from build123d import *

# Parameters (mm, degrees)
BOSS_EXTRUDE1_DEPTH                               = 20
CSK_FOR_3_FLAT_HEAD_MACHINE_SCREW_100_D           = 2.794
CSK_FOR_3_FLAT_HEAD_MACHINE_SCREW_100_DEPTH       = 20
CSK_FOR_3_FLAT_HEAD_MACHINE_SCREW_100_CSINK_D     = 5.0546
CSK_FOR_3_FLAT_HEAD_MACHINE_SCREW_100_CSINK_ANGLE = 100


with BuildPart() as part:
    # Sketch2 → Boss-Extrude1 (new body)
    with BuildSketch(Plane.XY):
        Polygon((-118.58, 345.487717935), (-863.58, 345.487717935), (-963.71, 209.828898833), (-963.71, -209.828898833), (-863.58, -345.487717935), (-118.58, -345.487717935), (0, -190.295), (0, 190.295), align=None)
    extrude(amount=BOSS_EXTRUDE1_DEPTH)

    # CSK for #3 Flat Head Machine Screw (100)1
    with Locations(Plane.XY.offset(20)):
        with Locations((-950.019491684, 82.340523551), (-950.019491684, 173.75453442), (-905.654330921, 268.705699397), (-803.58, 330.487717935), (-633.58, 330.487717935), (-455.480152545, 323.52139094), (-348.58, 330.487717935), (-178.58, 330.487717935), (-102.481993543, 302.529132765), (-48.296375955, 230.66872053), (-15.328698966, 110.295), (-15.328698966, -4.236762626), (-15.328698966, -110.295), (-50.699956706, -233.856324756), (-104.885574294, -305.716736991), (-178.58, -330.487717935), (-348.58, -330.487717935), (-455.480152545, -330.487717935), (-633.58, -330.487717935), (-803.58, -330.487717935), (-905.654330921, -268.716630557), (-950.019491684, -173.76546558), (-950.019491684, -82.351454711), (-950.019491684, -4.236762626)):
            CounterSinkHole(CSK_FOR_3_FLAT_HEAD_MACHINE_SCREW_100_D / 2, CSK_FOR_3_FLAT_HEAD_MACHINE_SCREW_100_CSINK_D / 2, depth=CSK_FOR_3_FLAT_HEAD_MACHINE_SCREW_100_DEPTH, counter_sink_angle=CSK_FOR_3_FLAT_HEAD_MACHINE_SCREW_100_CSINK_ANGLE)


solid = part.part
Check sheet for the modelled part. Datum: model origin and axes. Units: mm. Give positions to 0.01 mm unless a question says otherwise; leave off trailing zeros. Loops run counter-clockwise (first coordinate to the right, second up) from the corner with the lowest first, then second, coordinate; pieces in that order, holes last. Notation, with made-up numbers: M 31.5,53 L 44.5,53 A22 ccw 44.5,73 Z; hole C 25,9.5 d9. An arc over 180 degrees is marked long. Return JSON: item names as keys, results as strings. Group by question number.
1. Thickness scan on L1, parallel to Y at x = -632.5, z = 15.75; L2, parallel to X at y = -235, z = 12; L3, parallel to X at y = -277, z = 1.5. Record the ranges inside material, lowest first.
2. Cross-section at A-A on z = 10.75. State how many separate pieces and enclosed holes the cut face has, plus the area to 3 significant figures.
3. Go/stop test with flat-tipped pins: pin 1 (2 mm diameter, centred on x = -348.58, y = -330.49, fed in from -Z); pin 2 (3.5 mm diameter, centred on x = -50.7, y = -233.86, fed in from +Z); pin 3 (3.5 mm diameter, centred on x = -455.48, y = 323.52, fed in from +Z). Record where each tip stops, or that it passes through.
4. Cross-section at B-B on y = -282. Record the boundary of the cut face in (x, z), plus the area to 3 significant figures.
Return value:
{
 "1": {"L1": "-345.49 to -331.37, -329.6 to 329.6, 331.37 to 345.49", "L2": "-945.13 to -51.5, -49.9 to -34.16", "L3": "-914.13 to -66.25"},
 "2": {"separate pieces": "1", "enclosed holes": "24", "area": "634,000 mm^2"},
 "3": {"pin 1": "through", "pin 2": "z = 19.35", "pin 3": "z = 19.35"},
 "4": {"outline": "M -910.44,0 L -70.07,0 L -70.07,20 L -910.44,20 Z", "area": "16,800 mm^2"}
}
